Check sheet for the modelled part. Datum: model origin and axes. Units: mm. A direction names the side the tool comes from. Coordinates: 2 decimals unless noted, no trailing zeros. Write each loop counter-clockwise with the first axis right and the second up, starting at its lowest first coordinate (ties: lowest second). Pieces come first, ordered by that corner, then holes. Notation, with made-up numbers: M 2,34.5 L 9,34.5 A27 ccw 9,56.5 Z; hole C 50,-35 d6. An arc over 180 degrees is marked long. Answer as CSV lines item,"result". Start each with the question number.
Q1. Sectioned sample at A-A, the plane z = 18. Record the cut outline in (x, y) (1 decimal).
Q2. Mould release check, pull along Z, two halves, no side actions. Record for faces 1 (the flat face through (343.68, 8.17, 8.03)), 2 (the flat face through (174, 130.175, 30)), 3 (the flat face through (169, 64, 0)): pulls with the +Z half, pulls with the -Z half, needs draft (parallel to the pull), parting line crosses it, or undercut.
Q3. Thickness scan on line 1 along X through (y, z) = (6.5, 12); line 2 along Y through (x, z) = (235, 16) (1 decimal); line 3 along Z through (x, y) = (44, 1). Record the ranges inside material, lowest first. Write a range as from..to.
Q4. Depth check by flat-ended pin: pin 1 Ø3.5 at (y, z) = (122.24, 55.56) entering from +X; pin 2 Ø8 at (x, y) = (293, 15) entering from +Z; pin 3 Ø4 at (x, z) = (146.05, 61.91) entering from +Y; pin 4 Ø2.5 at (x, z) = (44.45, 61.91) entering from +Y. Enter the tip coordinate at first touch or a pass-through.
Q5. Sectioned sample at B-B, the plane y = 55. Record the cut outline in (x, z).
Q6. Access from +Z, -Z, +X, -X, +Y, -Y to the whole of each face (thin tool, end or side, straight path). Record for faces 4 (the flat face through (0, 8, 35)), 5 (the flat face through (344.487, 64, 12)), 6 (the flat face through (169, 128.588, 31)).
Q7. Sectioned sample at C-C, the plane x = 178. Record the cut outline in (y, z) (1 decimal), then the cut area to 3 significant figures.
from build123d import *

# Parameters (mm, degrees)
F1_DEPTH  = 342.9
F2_W      = 3.175
F2_H      = 12.7
F3_DEPTH  = 1.5945639921
F5_DEPTH  = 1.5875
F6_DEPTH  = 1.5875
F10_DEPTH = 1.5875
F11_R     = 1.5875
F12_DEPTH = 444.5
F13_R     = 1.5875
F14_DEPTH = 1.5875


# Not quite as in the source:
# - a feature names something its author has since deleted; it is built from what else it names


with BuildPart() as f1:
    # F0 (on Right) → F1 (new body)
    with BuildSketch(Plane.YZ):
        Polygon((0, 68.2625), (0, 0), (130.175, 0), (130.175, 58.7375), (129.0681220671, 71.3891726658), (127.4866629839, 71.2508129242), (128.5875, 58.7375), (128.5875, 1.5875), (1.5875, 1.5875), (1.5875, 68.2625), align=None)
    extrude(amount=F1_DEPTH)

    # F2 (on face) → F3 (cut, through all)
    with BuildSketch(Plane(origin=(0, 134.286004542, 11.7485030676), x_dir=(-1, 0, 0), z_dir=(0, 0.9961946981, 0.0871557427))):
        with Locations((-341.3125, 53.518487267)):
            Rectangle(F2_W, F2_H)
        with Locations((-1.5875, 53.518487267)):
            Rectangle(F2_W, F2_H)
    extrude(amount=-F3_DEPTH, mode=Mode.SUBTRACT)

    # F4 (on face) → F5 (join)
    with BuildSketch(Plane(origin=(0, 0, 0), x_dir=(0, -1, 0), z_dir=(-1, 0, 0))):
        Polygon((-128.5875, 58.5986117467), (-130.175, 58.7375), (-130.175, 0), (-128.5875, 1.6154517363), align=None)
        Polygon((-115.8881750797, 58.5986117466), (-130.175, 58.7375), (-128.5875, 58.5986117467), (-128.5875, 1.6154517363), (-115.8881750797, 14.538378661), align=None)
        Polygon((-115.6359343729, 14.2875), (-128.5595482637, 1.5875), (-1.6154517363, 1.5875), (-14.5390656271, 14.2875), align=None)
        Polygon((-14.2868249203, 14.538378661), (-1.5875, 1.6154517363), (-1.5875, 68.2625), (-14.2868249203, 68.2625), (-14.2868249203, 58.5986117466), align=None)
    extrude(amount=F5_DEPTH)


with BuildPart() as f6:
    # F6 (new): a face of the model
    f6_faces = [f1.part.faces().sort_by_distance(p)[0] for p in [
        (0, 129.2764111618, 0.7047010288),
    ]]
    extrude(f6_faces, amount=F6_DEPTH)


with BuildPart() as f1_1:
    add(f1.part)

    # F7: union F6
    add(f6.part)

    # F9 (on face) + F8 (on face) → F10 (join)
    with BuildSketch(Plane.YZ.offset(342.9)):
        Polygon((1.5875, 68.2625), (1.5875, 1.6154517363), (14.2868249203, 14.538378661), (14.2868249203, 58.5986117466), (14.2868249203, 68.2625), align=None)
        Polygon((115.8881750797, 14.538378661), (128.5875, 1.6154517363), (128.5875, 58.5986117467), (130.175, 58.7375), (115.8881750797, 58.5986117466), align=None)
        Polygon((128.5875, 1.6154517363), (130.175, 0), (130.175, 58.7375), (128.5875, 58.5986117467), align=None)
        Polygon((14.5390656271, 14.2875), (1.6154517363, 1.5875), (128.5595482637, 1.5875), (115.6359343729, 14.2875), align=None)
    with BuildSketch(Plane.YZ.offset(342.9)):
        Polygon((128.5875, 58.5986117467), (128.5875, 1.5875), (1.5875, 1.5875), (1.5875, 68.2625), (0, 68.2625), (0, 0), (130.175, 0), (130.175, 58.7375), align=None)
    extrude(amount=F10_DEPTH)

    # F11 (on face) → F12 (cut, symmetric)
    with BuildSketch(Plane.YZ):
        with Locations((7.9375, 55.5625)):
            Circle(F11_R)
        with Locations((7.9375, 27.0154517363)):
            Circle(F11_R)
        with Locations((26.9875, 7.9654517363)):
            Circle(F11_R)
        with Locations((122.2375, 55.5625)):
            Circle(F11_R)
        with Locations((122.2375, 27.0154517363)):
            Circle(F11_R)
        with Locations((103.1875, 7.9654517363)):
            Circle(F11_R)
    extrude(amount=F12_DEPTH, both=True, mode=Mode.SUBTRACT)

    # F13 (on face) → F14 (cut, through all)
    with BuildSketch(Plane.XZ):
        with Locations((44.45, 61.9125)):
            Circle(F13_R)
        with Locations((95.25, 61.9125)):
            Circle(F13_R)
        with Locations((146.05, 61.9125)):
            Circle(F13_R)
        with Locations((196.85, 61.9125)):
            Circle(F13_R)
        with Locations((247.65, 61.9125)):
            Circle(F13_R)
        with Locations((298.45, 61.9125)):
            Circle(F13_R)
    extrude(amount=-F14_DEPTH, mode=Mode.SUBTRACT)


solid = f1_1.part
Output:
1,outline,"M -1.6,0 L 344.5,0 L 344.5,14.3 L 342.9,14.3 L 342.9,1.6 L 0,1.6 L 0,14.3 L -1.6,14.3 Z; M -1.6,115.9 L 0,115.9 L 0,128.6 L 342.9,128.6 L 342.9,115.9 L 344.5,115.9 L 344.5,130.2 L -1.6,130.2 Z"
2,face 1,"undercut"
2,face 2,"needs draft"
2,face 3,"pulls with the -Z half"
3,line 1,"x = -1.59..0, 342.9..344.49"
3,line 2,"y = 0..1.6, 128.6..130.2"
3,line 3,"z = 0..60.39, 63.43..68.26"
4,pin 1,"stops at x = 344.49"
4,pin 2,"stops at z = 1.59"
4,pin 3,"stops at y = 130.07"
4,pin 4,"stops at y = 130.01"
5,outline,"M -1.59,0 L 344.49,0 L 344.49,14.29 L 342.9,14.29 L 342.9,1.59 L 0,1.59 L 0,14.29 L -1.59,14.29 Z"
6,face 4,"+Z"
6,face 5,"+Z, -Z, +X, +Y, -Y"
6,face 6,"none"
7,outline,"M 0,0 L 130.2,0 L 130.2,58.7 L 129.1,71.4 L 127.5,71.3 L 128.6,58.7 L 128.6,1.6 L 1.6,1.6 L 1.6,68.3 L 0,68.3 Z"
7,area,"423 mm^2"
